from build123d import *

# Parameters (mm, degrees)
F0_W          = 40
F0_H          = 40
F1_DEPTH      = 42.38128
F1_DEPTH_BACK = 7.75136
F2_W          = 11.914433
F2_H          = 33.472474
F3_DEPTH      = 52.48423
F4_SIZE       = 27.94
F5_R          = 8.402313
F6_DEPTH      = 40


with BuildPart() as f1:
    # F0 (on Front) → F1 (new body, two sides)
    with BuildSketch(Plane.XZ) as f1_sk:
        Rectangle(F0_W, F0_H)
    extrude(amount=F1_DEPTH)
    extrude(f1_sk.sketch, amount=-F1_DEPTH_BACK)

    # F2 (on face) → F3 (cut)
    with BuildSketch(Plane.XZ.offset(42.38128)):
        with Locations((-5.957216, 3.263763)):
            Rectangle(F2_W, F2_H)
        with Locations((5.957216, 3.263763)):
            Rectangle(F2_W, F2_H)
    extrude(amount=-F3_DEPTH, mode=Mode.SUBTRACT)

    # F4
    f4_edges = [f1.edges().sort_by_distance(p)[0] for p in [
        (-15.957216, -42.38128, 20),
        (15.957216, -42.38128, 20),
    ]]
    chamfer(f4_edges, length=F4_SIZE)

    # F5 (on face) → F6 (cut)
    with BuildSketch(Plane.YZ.offset(20)):
        with Locations((-6.598762, 0)):
            Circle(F5_R)
    extrude(amount=-F6_DEPTH, mode=Mode.SUBTRACT)


solid = f1.part
Input: part model. Units: mm. Frame: model coordinates. A direction names the side the tool comes from. Give positions to 0.01 mm unless a question says otherwise; leave off trailing zeros. Write each loop counter-clockwise with the first axis right and the second up, starting at its lowest first coordinate (ties: lowest second). Pieces come first, ordered by that corner, then holes. Notation, with made-up numbers: M 74.5,13 L 112.5,13 A34 ccw 112.5,43 Z; hole C -29,7.25 d2. An arc over 180 degrees is marked long. Write item = value, one per line. Start each with the question number.
1) Draft query along Z for faces 3 (the flat face through (11.914, -18, -1)), 4 (the flat face through (0, -18, -20)), 5 (the flat face through (16, -4, 20)), 6 (the cylindrical face through (16.01, -7.69, 8.33)). Return one class per face: +Z half, -Z half, draft (parallel to the pull), parting line (faces both ways), or undercut.
2) Cut plane A-A on z = -12.5. Return the cut outline in (x, y), then the cut area to 3 significant figures.
3) Cut plane C-C on z = -7. Return the cut outline in (x, y), then the cut area to 3 significant figures.
4) Cut plane D-D on y = -20. Return the cut outline in (x, z), then the cut area to 4 significant figures.
5) Material intervals for line 1 along X through (y, z) = (-33, -12); line 2 along Z through (x, y) = (-5, -39); line 3 along Y through (x, z) = (13.5, 6), sorted ascending. Write a range as [from, to].
6) Reachability of faces 1 (the flat face through (-16, -4, 20)), 2 (the flat face through (0, -18, -13.472)) from +Z, -Z, +X, -X, +Y, -Y: full face, straight path, thin tool, end or side. Return the list, or none.
7) First-contact query: pin 1 Ø3 at (x, y) = (-9, -32.5) entering from +Z; pin 2 Ø3 at (x, z) = (11, 5.5) entering from -Y. Flat tips, straight axial feed; report the tip coordinate or a pass-through.
8) Cut plane B-B on y = -11. Return the cut outline in (x, z).
Solved:
q1.face_3 = draft
q1.face_4 = -Z half
q1.face_5 = +Z half
q1.face_6 = undercut
q2.outline = M -20,-42.38 L -11.91,-42.38 L -11.91,7.75 L -20,7.75 Z; M 11.91,-42.38 L 20,-42.38 L 20,7.75 L 11.91,7.75 Z
q2.area = 811 mm2
q3.outline = M -20,-41.44 L -11.91,-41.44 L -11.91,-11.25 L -20,-11.25 Z; M -20,-1.95 L -11.91,-1.95 L -11.91,7.75 L -20,7.75 Z; M 11.91,-41.44 L 20,-41.44 L 20,-11.25 L 11.91,-11.25 Z; M 11.91,-1.95 L 20,-1.95 L 20,7.75 L 11.91,7.75 Z
q3.area = 645 mm2
q4.outline = M -20,-20 L 20,-20 L 20,14.44 L 11.91,14.44 L 11.91,-13.47 L -11.91,-13.47 L -11.91,14.44 L -20,14.44 Z
q4.area = 712.5 mm2
q5.line_1 = [-20, -11.91], [11.91, 20]
q5.line_2 = [-20, -13.47]
q5.line_3 = [-28.44, -12.48], [-0.72, 7.75]
q6.face_1 = +Z, +X, -X, +Y, -Y
q6.face_2 = +Z, +Y, -Y
q7.pin_1 = -13.47
q7.pin_2 = -30.13
q8.outline = M -20,-20 L 20,-20 L 20,-7.16 L 11.91,-7.16 L 11.91,-13.47 L -11.91,-13.47 L -11.91,-7.16 L -20,-7.16 Z; M -20,7.16 L -11.91,7.16 L -11.91,20 L -20,20 Z; M 11.91,7.16 L 20,7.16 L 20,20 L 11.91,20 Z
